```python
from build123d import *

# Parameters (mm, degrees)
BOSS_EXTRUDE1_DEPTH  = 38.1
SKETCH7_W            = 101.6
SKETCH7_H            = 20.32
BOSS_EXTRUDE2_DEPTH  = 44.45
BOSS_EXTRUDE8_DEPTH  = 12.7
SKETCH8_W            = 22.86
SKETCH8_H            = 13.208
CUT_EXTRUDE1_DEPTH   = 20.32
SKETCH9_R            = 4.826
CUT_EXTRUDE2_DEPTH   = 114.3
LPATTERN1_COUNT      = 3
LPATTERN1_PITCH      = 34.067332164
LPATTERN1_COUNT_DIR2 = 2
LPATTERN1_PITCH_DIR2 = 100.965


with BuildPart() as part:
    # Sketch1 → Boss-Extrude1 (new body)
    with BuildSketch(Plane.XY):
        with BuildLine():
            Line((-50.8, 0), (50.8, 0))
            Line((50.8, 0), (50.8, 20.32))
            Line((50.8, 20.32), (36.83, 20.32))
            ThreePointArc((36.83, 20.32), (35.714076836, 15.394076836), (32.584204897, 11.43))
            Line((32.584204897, 11.43), (18.215795103, 11.43))
            ThreePointArc((18.215795103, 11.43), (15.085923164, 15.394076836), (13.97, 20.32))
            Line((13.97, 20.32), (-13.97, 20.32))
            ThreePointArc((-13.97, 20.32), (-15.085923164, 15.394076836), (-18.215795103, 11.43))
            Line((-18.215795103, 11.43), (-32.584204897, 11.43))
            ThreePointArc((-32.584204897, 11.43), (-35.714076836, 15.394076836), (-36.83, 20.32))
            Line((-36.83, 20.32), (-50.8, 20.32))
            Line((-50.8, 20.32), (-50.8, 0))
        make_face()
    extrude(amount=BOSS_EXTRUDE1_DEPTH)

    # Sketch7 → Boss-Extrude2 (add)
    with BuildSketch(Plane.XY.offset(38.1)):
        with Locations((0, 10.16)):
            Rectangle(SKETCH7_W, SKETCH7_H)
    extrude(amount=BOSS_EXTRUDE2_DEPTH)

    # Sketch20 → Boss-Extrude8 (add)
    with BuildSketch(Plane(origin=(50.8, 0, 0), x_dir=(0, 0, -1), z_dir=(1, 0, 0))):
        Polygon((-50.8, 0), (0, 0), (0, 7.112), (-50.8, 7.112), (-50.8, 20.32), (-82.55, 20.32), (-82.55, 3.874334441), (-82.55, 0), align=None)
    extrude(amount=BOSS_EXTRUDE8_DEPTH)

    # Sketch8 → Cut-Extrude1 (cut)
    with BuildSketch(Plane(origin=(0, 20.32, 0), x_dir=(1, 0, 0), z_dir=(0, 1, 0))):
        with Locations((-25.4, -44.704)):
            Rectangle(SKETCH8_W, SKETCH8_H)
        with Locations((25.4, -44.704)):
            Rectangle(SKETCH8_W, SKETCH8_H)
    extrude(amount=-CUT_EXTRUDE1_DEPTH, mode=Mode.SUBTRACT)

    # Sketch5 → #10 (0.1935) Diameter Hole1 (revolve, cut)
    with BuildSketch(Plane(origin=(-43.815, 20.32, 8.89), x_dir=(0, 0, 1), z_dir=(1, 0, 0))):
        Polygon((0, 0), (0, 25.4), (2.45745, 23.923415072), (2.45745, 0), align=None)
    f_10_0_1935_diameter_hole1 = revolve(axis=Axis((-43.815, 26.67, 8.89), (0, -1, 0)), mode=Mode.SUBTRACT)

    # Sketch9 → Cut-Extrude2 (cut)
    with BuildSketch(Plane.ZY.offset(50.8)):
        with Locations((66.675, 20.447)):
            Circle(SKETCH9_R)
    extrude(amount=-CUT_EXTRUDE2_DEPTH, mode=Mode.SUBTRACT)

    # LPattern1: 10 _0.1935_ Diameter Hole1 3 × 2
    with Locations(*[(j * LPATTERN1_PITCH_DIR2, 0, i * LPATTERN1_PITCH) for i in range(LPATTERN1_COUNT) for j in range(LPATTERN1_COUNT_DIR2) if (i, j) != (0, 0)]):
        add(f_10_0_1935_diameter_hole1, mode=Mode.SUBTRACT)


solid = part.part
```
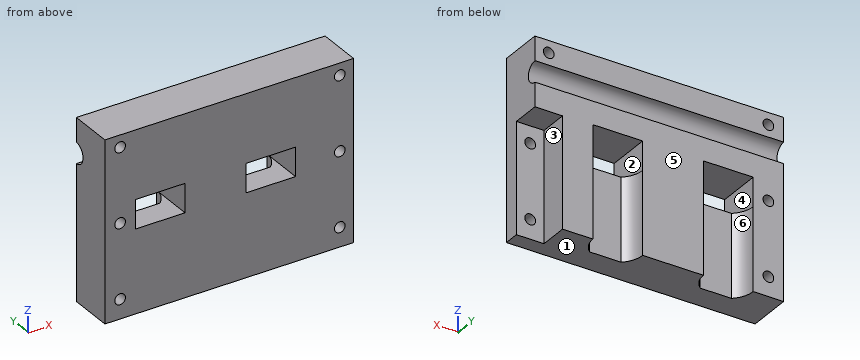
Source: CAD feature listing. Evaluate the final solid. Frame: model axes, mm. Face numbers are marked on the shaded views. A direction names the side the tool comes from. Coordinates: 2 decimals unless noted, no trailing zeros. Write each loop counter-clockwise with the first axis right and the second up, starting at its lowest first coordinate (ties: lowest second). Pieces come first, ordered by that corner, then holes. Notation, with made-up numbers: (0, -18) - (38, -18) arc R25 cw to (38, 17) - close; hole circle Ø8 at (26.5, -31). An arc over 180 degrees is marked (long way). Answer as a JSON object with one key per item and string values.
Q1. Section query D-D, the plane x = 57.15. Output: boundary loops of the cut face in (y, z) (3 decimals), plus the area to 3 significant figures.
Ans:
{"outline": "(0, 0) - (7.112, 0) - (7.112, 6.433) - (0, 6.433) - close; (0, 11.347) - (7.112, 11.347) - (7.112, 40.5) - (0, 40.5) - close; (0, 45.415) - (7.112, 45.415) - (7.112, 50.8) - (20.32, 50.8) - (20.32, 61.851) arc R4.826 cw to (20.32, 71.499) - (20.32, 74.567) - (0, 74.567) - close; (0, 79.482) - (20.32, 79.482) - (20.32, 82.55) - (0, 82.55) - close", "area": "801 mm2"}
Q2. Section query C-C, the plane z = 19. Output: boundary loops of the cut face in (x, y), plus the area to 3 significant figures.
Ans:
{"outline": "(-50.8, 0) - (63.5, 0) - (63.5, 7.11) - (50.8, 7.11) - (50.8, 20.32) - (36.83, 20.32) arc R11.43 cw to (32.58, 11.43) - (18.22, 11.43) arc R11.43 cw to (13.97, 20.32) - (-13.97, 20.32) arc R11.43 cw to (-18.22, 11.43) - (-32.58, 11.43) arc R11.43 cw to (-36.83, 20.32) - (-50.8, 20.32) - close", "area": "1,790 mm2"}
Q3. Draft query along X for the marked faces 1, 2 and 3. Return one class per face: released by +X, released by -X, zero draft, split by the parting line, or undercut.
Ans:
{"face 1": "zero draft", "face 2": "undercut", "face 3": "released by +X"}
Q4. Section query B-B, the plane z = 8.89. Output: boundary loops of the cut face in (x, y).
Ans:
{"outline": "(-50.8, 0) - (-46.27, 0) - (-46.27, 20.32) - (-50.8, 20.32) - close; (-41.36, 0) - (54.69, 0) - (54.69, 7.11) - (50.8, 7.11) - (50.8, 20.32) - (36.83, 20.32) arc R11.43 cw to (32.58, 11.43) - (18.22, 11.43) arc R11.43 cw to (13.97, 20.32) - (-13.97, 20.32) arc R11.43 cw to (-18.22, 11.43) - (-32.58, 11.43) arc R11.43 cw to (-36.83, 20.32) - (-41.36, 20.32) - close; (59.61, 0) - (63.5, 0) - (63.5, 7.11) - (59.61, 7.11) - close"}
Q5. Section query A-A, the plane x = 24.5. Output: boundary loops of the cut face in (y, z) (3 decimals), plus the area to 3 significant figures.
Ans:
{"outline": "(0, 0) - (11.43, 0) - (11.43, 38.1) - (0, 38.1) - close; (0, 51.308) - (20.32, 51.308) - (20.32, 61.851) arc R4.826 cw to (20.32, 71.499) - (20.32, 82.55) - (0, 82.55) - close", "area": "1,030 mm2"}
Q6. Material intervals for line 1 (X direction, y = 4.25, z = 8.89); line 2 (X direction, y = 16, z = 46.5); line 3 (Z direction, x = 16, y = 6), sorted ascending. Write a range as [from, to].
Ans:
{"line 1": "x = [-50.8, -46.27], [-41.36, 54.69], [59.61, 63.5]", "line 2": "x = [-50.8, -36.83], [-13.97, 13.97], [36.83, 50.8]", "line 3": "z = [0, 38.1], [51.31, 82.55]"}
Q7. First-contact query: pin 1 Ø4 at (y, z) = (12, 43) entering from +X; pin 2 Ø16 at (x, z) = (24.5, 25.5) entering from +Y; pin 3 Ø7 at (x, z) = (-24, 15) entering from +Y. Flat tips, straight axial feed; report the tip coordinate or a pass-through.
Ans:
{"pin 1": "stops at x = 50.8", "pin 2": "stops at y = 13.15", "pin 3": "stops at y = 11.43"}
Q8. Set-up query: the marked faces 4, 5 and 6. Return all of +Z, -Z, +X, -X, +Y, -Y with unobstructed straight access to the full face (end or side cutting, diameter ignored); none if empty.
Ans:
{"face 4": "+Y, -Y", "face 5": "+Z, -Z, +X, -X, +Y", "face 6": "-Z, +Y"}
